CAD build for the part. Positions are in the model's coordinates, mm. A direction names the side the tool comes from. Give positions to 0.01 mm unless a question says otherwise; leave off trailing zeros. Write each loop counter-clockwise with the first axis right and the second up, starting at its lowest first coordinate (ties: lowest second). Pieces come first, ordered by that corner, then holes. Notation, with made-up numbers: (72.25, 84.5) - (97.25, 84.5) arc R4 ccw to (97.25, 91.5) - close; hole circle Ø11 at (-14.5, 4.25). An arc over 180 degrees is marked (long way). Answer as a JSON object with one key per item and string values.
from build123d import *

# Parameters (mm, degrees)
SKETCH1_R           = 100
BOSS_EXTRUDE1_DEPTH = 600
SKETCH2_W           = 50
SKETCH2_H           = 50
CUT_EXTRUDE1_DEPTH  = 150
SKETCH3_W           = 50
SKETCH3_H           = 50
CUT_EXTRUDE2_DEPTH  = 150


with BuildPart() as part:
    # Sketch1 → Boss-Extrude1 (new body)
    with BuildSketch(Plane.XY):
        Circle(SKETCH1_R)
    extrude(amount=-BOSS_EXTRUDE1_DEPTH)

    # Sketch2 → Cut-Extrude1 (cut)
    with BuildSketch(Plane.XY):
        with Locations((0, 86.4)):
            Rectangle(SKETCH2_W, SKETCH2_H)
    extrude(amount=-CUT_EXTRUDE1_DEPTH, mode=Mode.SUBTRACT)

    # Sketch3 → Cut-Extrude2 (cut)
    with BuildSketch(Plane(origin=(0, 0, -600), x_dir=(-1, 0, 0), z_dir=(0, 0, -1))):
        with Locations((0, 86.4)):
            Rectangle(SKETCH3_W, SKETCH3_H)
    extrude(amount=-CUT_EXTRUDE2_DEPTH, mode=Mode.SUBTRACT)


solid = part.part
(1) Saw through at C-C, the plane z = -422. Give the cut face in (x, y).
Answer key:
{"outline": "circle Ø200 at (0, 0)"}
(2) Probe L1, parallel to Y at x = -5, z = -177.5; L2, parallel to X at y = -81.5, z = -368.5; L3, parallel to X at y = 69, z = -388. List the from-to ranges inside material, lowest first. Write a range as [from, to].
Answer key:
{"L1": "y = [-99.87, 99.87]", "L2": "x = [-57.95, 57.95]", "L3": "x = [-72.38, 72.38]"}
(3) Saw through at A-A, the plane x = 0. Give the cut face in (y, z), and give its area (3 significant figures).
Answer key:
{"outline": "(-100, -600) - (61.4, -600) - (61.4, -450) - (100, -450) - (100, -150) - (61.4, -150) - (61.4, 0) - (-100, 0) - close", "area": "108,000 mm²"}
(4) Flat gauge pins, fed straight in: P1, Ø17.5, axis at y = 84, z = -48, coming from the -X side; P2, Ø1, axis at y = 35, z = -74.5, coming from the +X side; P3, Ø17.5, axis at y = 80, z = -85.5, coming from the +X side. Where does each tip first touch, or does it go through?
Answer key:
{"P1": "stops at x = -65.86", "P2": "stops at x = 93.86", "P3": "stops at x = 70.17"}
(5) Saw through at D-D, the plane z = -118.5. Give the cut face in (x, y).
Answer key:
{"outline": "(-25, 61.4) - (-25, 96.82) arc R100 ccw (long way) to (25, 96.82) - (25, 61.4) - close"}
(6) 3-axis set-ups, long thin cutter, end or side, ignore diameter. For faces 4 (the face through (-1, 0, 0)), 5 (the face through (-25, 79, -74)), 6 (the face through (0, 81, -450)): which of +Z, -Z, +X, -X, +Y, -Y reach the whole face in a straight line?
Answer key:
{"face 4": "+Z, +X, -X, +Y, -Y", "face 5": "+Z, +Y", "face 6": "-Z, +Y"}
(7) Pull direction X, two halves, no side cores. Call faces 1 (the face through (25, 79, -74)), 2 (the face through (-1, 0, -600)), 3 (the face through (46.14, -88.72, -295.8)): pulls with the +X half, pulls with the -X half, needs draft (parallel to the pull), parting line crosses it, or undercut.
Answer key:
{"face 1": "undercut", "face 2": "needs draft", "face 3": "parting line crosses it"}
(8) Saw through at B-B, the plane y = 86. Give the cut face in (x, z).
Answer key:
{"outline": "(-51.03, -600) - (-25, -600) - (-25, -450) - (25, -450) - (25, -600) - (51.03, -600) - (51.03, 0) - (25, 0) - (25, -150) - (-25, -150) - (-25, 0) - (-51.03, 0) - close"}
